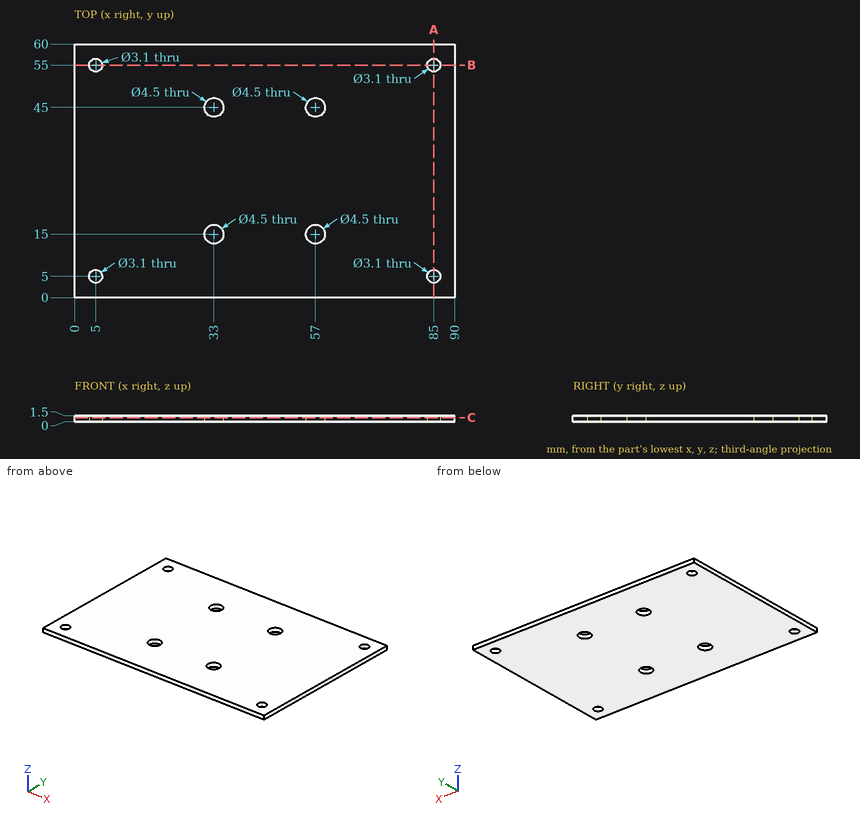
The drawing under review shows one solid part. Ordinate dimensions are in mm from its lowest x, y, z. Round coordinates to 2 decimals unless told otherwise and drop trailing zeros. Write each loop counter-clockwise with the first axis right and the second up, starting at its lowest first coordinate (ties: lowest second). Pieces come first, ordered by that corner, then holes. Notation, with made-up numbers: M 46.5,36 L 85.5,36 A17 cw 85.5,45 Z; hole C 66,78 d1. An arc over 180 degrees is marked long. One line per item, written item: value. Start each with the question number.
(1) We need section A-A (x = 85). Give the boundary of the cut face in (y, z).
(2) We need section B-B (y = 55). Give the boundary of the cut face in (x, z), and give its area (3 significant figures).
(3) Wall thickness on line 1 (X direction, y = 45, z = 0.65); line 2 (X direction, y = 5, z = 0.45); line 3 (Y direction, x = 85, z = 0.65): over which ranges is each line inside the solid? List them lowest first.
(4) We need section C-C (z = 1.05). Count the separate pieces of the cut face and the enclosed holes in it, and give its area (3 significant figures).
Result:
1. outline: M 0,0 L 3.45,0 L 3.45,1.5 L 0,1.5 Z; M 6.55,0 L 53.45,0 L 53.45,1.5 L 6.55,1.5 Z; M 56.55,0 L 60,0 L 60,1.5 L 56.55,1.5 Z
2. outline: M 0,0 L 3.45,0 L 3.45,1.5 L 0,1.5 Z; M 6.55,0 L 83.45,0 L 83.45,1.5 L 6.55,1.5 Z; M 86.55,0 L 90,0 L 90,1.5 L 86.55,1.5 Z
2. area: 126 mm²
3. line 1: 0 to 30.75, 35.25 to 54.75, 59.25 to 90
3. line 2: 0 to 3.45, 6.55 to 83.45, 86.55 to 90
3. line 3: 0 to 3.45, 6.55 to 53.45, 56.55 to 60
4. separate pieces: 1
4. enclosed holes: 8
4. area: 5,310 mm²
